```python
from build123d import *

# Parameters (mm, degrees)
F1_DEPTH = 500
F2_W     = 35
F2_H     = 25
F3_DEPTH = 25
F4_R     = 5


with BuildPart() as f1:
    # F0 (on Right) → F1 (new body)
    with BuildSketch(Plane.YZ):
        with BuildLine():
            Line((0, 75), (0, 0))
            Line((0, 0), (9.5, 0))
            Line((9.5, 0), (9.5, 57))
            ThreePointArc((9.5, 57), (13.014719, 65.485281), (21.5, 69))
            Line((21.5, 69), (128.5, 69))
            ThreePointArc((128.5, 69), (136.985281, 65.485281), (140.5, 57))
            Line((140.5, 57), (140.5, 0))
            Line((140.5, 0), (150, 0))
            Line((150, 0), (150, 75))
            Line((150, 75), (0, 75))
        make_face()
    extrude(amount=F1_DEPTH)

    # F2 (on Front) → F3 (cut)
    with BuildSketch(Plane.XZ):
        with Locations((482.5, 62.5)):
            Rectangle(F2_W, F2_H)
    extrude(amount=-F3_DEPTH, mode=Mode.SUBTRACT)

    # F4
    f4_edges = [f1.edges().sort_by_distance(p)[0] for p in [
        (465, 25, 72),
        (465, 4.75, 50),
    ]]
    fillet(f4_edges, radius=F4_R)

    # F5: F1 across plane


with BuildPart() as f1_1:
    add(f1.part)
    add(f1.part.mirror(Plane.YZ))


solid = f1_1.part
```
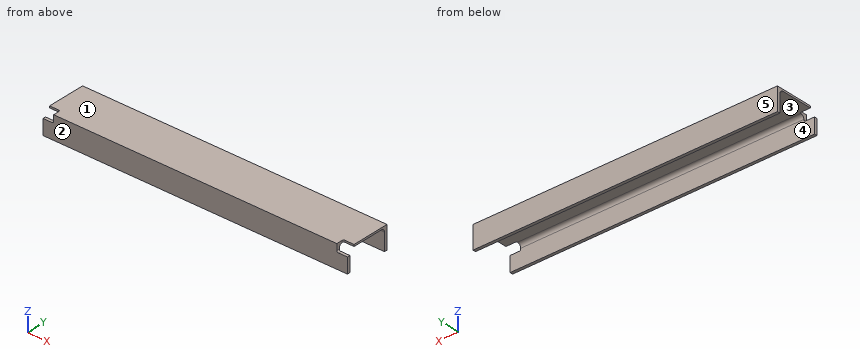
Source: CAD feature listing. Evaluate the final solid. Frame: model axes, mm. Face numbers are marked on the shaded views. A direction names the side the tool comes from. Give positions to 0.01 mm unless a question says otherwise; leave off trailing zeros. Write each loop counter-clockwise with the first axis right and the second up, starting at its lowest first coordinate (ties: lowest second). Pieces come first, ordered by that corner, then holes. Notation, with made-up numbers: (82.5, 81.25) - (112.5, 81.25) arc R10 ccw to (112.5, 94.25) - close; hole circle Ø9 at (26.25, 8.25). An arc over 180 degrees is marked (long way). One line per item, written item: value. Start each with the question number.
Q1. Set-up query: the marked faces 4 and 5. Return all of +Z, -Z, +X, -X, +Y, -Y with unobstructed straight access to the full face (end or side cutting, diameter ignored); none if empty.
Q2. Material intervals for probe 1 along Y at (x, z) = (-264.5, 25); probe 2 along Z at (x, y) = (234.5, 40.5); probe 3 along Y at (x, z) = (-246, 64), sorted ascending. Write a range as from..to.
Q3. First-contact query: pin 1 Ø3 at (x, z) = (205.5, 63) entering from -Y; pin 2 Ø5 at (x, y) = (-78, 108) entering from -Z; pin 3 Ø7.5 at (x, y) = (479, 5) entering from +Z; pin 4 Ø3 at (x, z) = (490.5, 72.5) entering from -Y. Flat tips, straight axial feed; report the tip coordinate or a pass-through.
Q4. Draft query along Y for the marked faces 1, 2 and 3. Return one class per face: +Y half, -Y half, draft (parallel to the pull), parting line (faces both ways), or undercut.
Q5. Section query B-B, the plane x = 163. Return the cut outline in (y, z), then the cut area to 3 significant figures.
Q6. Section query C-C, the plane y = 114. Return the cut outline in (x, z).
Q7. Section query A-A, the plane z = 12.5. Return the cut outline in (x, y), then the cut area to 3 significant figures.
Answer:
1. face 4: -Z, +X, -X
1. face 5: +Z, -Z, +X, -X, +Y
2. probe 1: y = 0..9.5, 140.5..150
2. probe 2: z = 69..75
2. probe 3: y = 0..11.75, 138.25..150
3. pin 1: stops at y = 0
3. pin 2: stops at z = 69
3. pin 3: stops at z = 50
3. pin 4: stops at y = 25
4. face 1: draft
4. face 2: -Y half
4. face 3: undercut
5. outline: (0, 0) - (9.5, 0) - (9.5, 57) arc R12 cw to (21.5, 69) - (128.5, 69) arc R12 cw to (140.5, 57) - (140.5, 0) - (150, 0) - (150, 75) - (0, 75) - close
5. area: 2,270 mm2
6. outline: (-500, 69) - (500, 69) - (500, 75) - (-500, 75) - close
7. outline: (-500, 0) - (500, 0) - (500, 9.5) - (-500, 9.5) - close; (-500, 140.5) - (500, 140.5) - (500, 150) - (-500, 150) - close
7. area: 19,000 mm2
